Work out the finished part from the listing and answer in its coordinate system (mm). Face numbers are marked on the shaded views. A direction names the side the tool comes from. Coordinates: 2 decimals unless noted, no trailing zeros. Order: outer loops, then holes, each group sorted by start corner. A loop starts at its lowest first (then second) coordinate and runs counter-clockwise, first axis right, second up. Notation, with made-up numbers: M -25,36 L -9,36 A17 ccw -9,56 Z; hole C 16.5,24 d1. An arc over 180 degrees is marked long. Use a Markdown table: item, result.
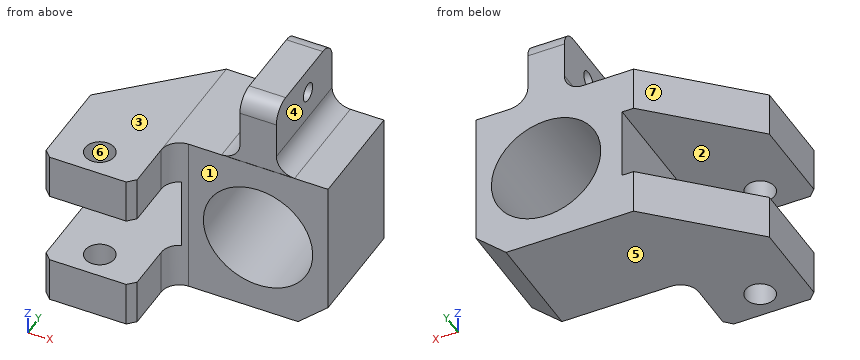
from build123d import *

# Parameters (mm, degrees)
EXTRUDE_1_DEPTH       = 30
SKETCH_2_R            = 15
CUT_EXTRUDE_2_DEPTH   = 45.532745299
EXTRUDE_3_DEPTH       = 44.84276
CUT_EXTRUDE_START     = 70
SKETCH_3_W            = 44.656689001
SKETCH_3_H            = 20
CUT_EXTRUDE_1_DEPTH   = 130
SKETCH_7_R            = 3.999999997
CUT_EXTRUDE_2_2_DEPTH = 73.895417278
FILLET_1_R            = 5
CHAMFER_5_SIZE        = 2
SKETCH_8_W            = 10
SKETCH_8_H            = 29.95730412
EXTRUDE_4_DEPTH       = 20
FILLET_2_R            = 5
SKETCH_10_R           = 2.5
CUT_EXTRUDE_3_DEPTH   = 75.906399488


with BuildPart() as part:
    # Эскиз1 → Вытянуть1 (new body)
    with BuildSketch(Plane(origin=(0, 0, 0), x_dir=(1, 0, 0), z_dir=(0, 1, 0))):
        Polygon((-24.019063342, 22.5), (10.980936658, 22.5), (19.22346273, 15), (19.22346273, -22.342761837), (-24.019063342, -22.342761837), align=None)
    extrude(amount=EXTRUDE_1_DEPTH)

    # Эскиз2 → Cut-Extrude 2 (cut, through all)
    with BuildSketch(Plane(origin=(0, 30, 0), x_dir=(1, 0, 0), z_dir=(0, 1, 0))):
        with Locations(Location((0, 0, 0), (0, 0, 270))):
            Circle(SKETCH_2_R)
    extrude(amount=-CUT_EXTRUDE_2_DEPTH, mode=Mode.SUBTRACT)

    # Эскиз6 → Вытянуть3 (add)
    with BuildSketch(Plane(origin=(0, 0, -22.5), x_dir=(-1, 0, 0), z_dir=(0, 0, -1))):
        Polygon((24.019063342, -19.927530698), (24.019063342, 30), (49.019063342, 6.012561534), (49.019063342, -19.927530698), align=None)
    extrude(amount=-EXTRUDE_3_DEPTH)

    # Эскиз3 → Вырез-Вытянуть1 (cut)
    with BuildSketch(Plane(origin=(0, 30, 0), x_dir=(1, 0, 0), z_dir=(0, 1, 0)).offset(CUT_EXTRUDE_START)):
        with Locations((-43.210774099, 0)):
            Rectangle(SKETCH_3_W, SKETCH_3_H)
    extrude(amount=-CUT_EXTRUDE_1_DEPTH, mode=Mode.SUBTRACT)

    # Эскиз7 → Cut-Extrude 2 2 (cut, through all)
    with BuildSketch(Plane(origin=(0, 0, -22.5), x_dir=(-1, 0, 0), z_dir=(0, 0, -1))):
        with Locations((37.000000002, -12.578306382)):
            Circle(SKETCH_7_R)
    extrude(amount=-CUT_EXTRUDE_2_2_DEPTH, mode=Mode.SUBTRACT)

    # Скругление1
    # the kernel refuses this fillet: 5 mm, written as the material it adds along each edge
    with BuildSketch(Plane(origin=(-24.019063342, 0, 34.84276), x_dir=(1, 0, 0), z_dir=(0, 0, -1))) as fillet_1_piece_1_section:
        with BuildLine():
            CenterArc((FILLET_1_R, FILLET_1_R), FILLET_1_R, 180, 90)
            Line((0, FILLET_1_R), (0, 0))
            Line((0, 0), (FILLET_1_R, 0))
        make_face()
    fillet_1_piece_1 = extrude(amount=24.84276, mode=Mode.PRIVATE)
    fillet_1_piece_1 = split(fillet_1_piece_1, bisect_by=Plane(origin=(-20.42000997, -0.107354451, 22.342761837), z_dir=(0, 0, -1)), keep=Keep.TOP, mode=Mode.PRIVATE)
    add(fillet_1_piece_1)
    with BuildSketch(Plane(origin=(-24.019063342, 0, 22.34276), x_dir=(1, 0, 0), z_dir=(0, 0, -1))) as fillet_1_piece_2_section:
        with BuildLine():
            CenterArc((FILLET_1_R, FILLET_1_R), FILLET_1_R, 180, 90)
            Line((0, FILLET_1_R), (0, 0))
            Line((0, 0), (FILLET_1_R, 0))
        make_face()
    fillet_1_piece_2 = extrude(amount=24.84276, mode=Mode.PRIVATE)
    fillet_1_piece_2 = split(fillet_1_piece_2, bisect_by=Plane(origin=(-20.882429598, -0.107354451, 3.75), z_dir=(1, 0, 0)), keep=Keep.TOP, mode=Mode.PRIVATE)
    add(fillet_1_piece_2)
    with BuildSketch(Plane(origin=(-24.019063342, 0, 2.5), x_dir=(1, 0, 0), z_dir=(0, 0, -1))) as fillet_1_piece_3_section:
        with BuildLine():
            CenterArc((FILLET_1_R, FILLET_1_R), FILLET_1_R, 180, 90)
            Line((0, FILLET_1_R), (0, 0))
            Line((0, 0), (FILLET_1_R, 0))
        make_face()
    fillet_1_piece_3 = extrude(amount=25, mode=Mode.PRIVATE)
    fillet_1_piece_3 = split(fillet_1_piece_3, bisect_by=Plane(origin=(-20.882429598, -0.107354451, -3.75), z_dir=(1, 0, 0)), keep=Keep.TOP, mode=Mode.PRIVATE)
    add(fillet_1_piece_3)
    with BuildSketch(Plane(origin=(-24.019063342, 0, -10), x_dir=(1, 0, 0), z_dir=(0, 0, -1))) as fillet_1_piece_4:
        with BuildLine():
            CenterArc((FILLET_1_R, FILLET_1_R), FILLET_1_R, 180, 90)
            Line((0, FILLET_1_R), (0, 0))
            Line((0, 0), (FILLET_1_R, 0))
        make_face()
    extrude(amount=12.5)
    # the kernel refuses this fillet: 5 mm, written as the material it takes off along each edge

    # Фаска5
    chamfer_5_edges = [part.edges().sort_by_distance(p)[0] for p in [
        (-49.019063342, -19.927530698, 16.17138),
        (-24.019063342, -19.927530698, 16.17138),
        (-24.019063342, -19.927530698, -16.25),
        (-49.019063342, -19.927530698, -16.25),
    ]]
    chamfer(chamfer_5_edges, length=CHAMFER_5_SIZE)

    # Эскиз8 → Вытянуть4 (add)
    with BuildSketch(Plane.XY.offset(22.342761837)):
        with Locations((0, 15.02134794)):
            Rectangle(SKETCH_8_W, SKETCH_8_H)
    extrude(amount=EXTRUDE_4_DEPTH)

    # Скругление2
    fillet_2_edges = [part.edges().sort_by_distance(p)[0] for p in [
        (0, 30, 42.342761837),
        (0, 0.04269588, 42.342761837),
        (-5, 15.02134794, 22.342761837),
        (5, 15.02134794, 22.342761837),
    ]]
    fillet(fillet_2_edges, radius=FILLET_2_R)

    # Эскиз10 → Вырез-Вытянуть3 (cut, through all)
    with BuildSketch(Plane(origin=(5, 0, 0), x_dir=(0, 0, -1), z_dir=(1, 0, 0))):
        with Locations(Location((-35.296798075, 17.052712081, 0), (0, 0, 90))):
            Circle(SKETCH_10_R)
    extrude(amount=-CUT_EXTRUDE_3_DEPTH, mode=Mode.SUBTRACT)


solid = part.part
(1) A cutting plane is placed at D-D (z = 11.5). Determine the outline of the cut face in (x, y).
Conclusion:
| item | result |
|---|---|
| outline | M -49.02,-17.93 L -47.02,-19.93 L -26.02,-19.93 L -24.02,-17.93 L -24.02,-5 A5 cw -19.02,0 L -9.63,0 L -9.63,30 L -24.02,30 L -49.02,6.01 Z; M 9.63,0 L 19.22,0 L 19.22,30 L 9.63,30 Z; hole C -37,-12.58 d8 |
(2) Given P1, Ø1, axis at y = 0.5, z = -0.5, coming from the -X side; P2, Ø6.5, axis at y = 17.05, z = 35.3, coming from the -X side; P3, Ø14, axis at y = -12, z = -18.5, coming from the +X side, each flat-ended and moving along its own axis, determine where each tip first touches the part or whether it passes through.
Conclusion:
| item | result |
|---|---|
| P1 | x = -20.88 |
| P2 | x = -5 |
| P3 | x = -24.02 |
(3) Which of the six approach directions +Z, -Z, +X, -X, +Y, -Y give full straight-line access (tool end or side, diameter ignored) to the marked faces 1, 2, 3 and 4?
Conclusion:
| item | result |
|---|---|
| face 1 | +Z, -Z, +X, -Y |
| face 2 | -X, +Y, -Y |
| face 3 | +Z, -X, +Y, -Y |
| face 4 | +Z, +X, +Y, -Y |
(4) Determine the mould class of the marked faces 5, 6 and 7 for opening direction X: pulls with the +X half, pulls with the -X half, needs draft (parallel to the pull), parting line crosses it, or undercut.
Conclusion:
| item | result |
|---|---|
| face 5 | needs draft |
| face 6 | undercut |
| face 7 | pulls with the -X half |
(5) A cutting plane is placed at B-B (x = 0). Determine the outline of the cut face in (y, z), then the cut area to 3 significant figures.
Conclusion:
| item | result |
|---|---|
| outline | M 0,-22.5 L 30,-22.5 L 30,-15 L 0,-15 Z; M 0,15 L 30,15 L 30,37.34 A5 ccw 25,42.34 L 5.04,42.34 A5 ccw 0.04,37.34 L 0.04,22.34 L 0,22.34 Z; hole C 17.05,35.3 d5 |
| area | 1,010 mm2 |
(6) Straight lines are drawn through the part: L1, parallel to Z at x = -24.5, y = 24; L2, parallel to X at y = 5, z = 0; L3, parallel to X at y = 20, z = 38. For each, find the intervals that lie inside material, in ascending order.
Conclusion:
| item | result |
|---|---|
| L1 | -22.5 to -10, 10 to 22.34 |
| L2 | -20.88 to -15, 15 to 19.22 |
| L3 | -5 to 5 |
(7) A cutting plane is placed at A-A (z = 0). Determine the outline of the cut face in (x, y), then the cut area to 3 significant figures.
Conclusion:
| item | result |
|---|---|
| outline | M -20.88,-0.36 A5 cw -19.02,0 L -15,0 L -15,30 L -20.88,30 Z; M 15,0 L 19.22,0 L 19.22,30 L 15,30 Z |
| area | 303 mm2 |
